```python
from build123d import *

# Parameters (mm, degrees)
F2_W     = 914.4
F2_H     = 457.2
F3_DEPTH = 57.15
F5_DEPTH = 53.975
F6_DEPTH = 57.15


# Not quite as in the source:
# - a length typed as a fraction of an inch, garbled in the dataset ("3 / 203.2 mm" for 3/8 in), is restored


with BuildPart() as f3:
    # F2 (on Top) → F3 (new body)
    with BuildSketch(Plane.XY):
        with Locations((457.2, 228.6)):
            Rectangle(F2_W, F2_H)
    extrude(amount=F3_DEPTH)

    # F4 (on face) → F5 (cut)
    with BuildSketch(Plane.XY.offset(57.15)):
        with BuildLine():
            ThreePointArc((47.625, 23.8125), (44.4270821412, 11.8930134592), (35.692262203, 3.175))
            Line((35.692262203, 3.175), (878.707737797, 3.175))
            ThreePointArc((878.707737797, 3.175), (873.749519773, 40.650480227), (911.225, 35.692262203))
            Line((911.225, 35.692262203), (911.225, 421.507737797))
            ThreePointArc((911.225, 421.507737797), (873.749519773, 416.549519773), (878.707737797, 454.025))
            Line((878.707737797, 454.025), (35.692262203, 454.025))
            ThreePointArc((35.692262203, 454.025), (44.4270821412, 445.3069865408), (47.625, 433.3875))
            ThreePointArc((47.625, 433.3875), (29.9608610621, 410.3824394154), (3.175, 421.507737797))
            Line((3.175, 421.507737797), (3.175, 35.692262203))
            ThreePointArc((3.175, 35.692262203), (29.9608610621, 46.8175605846), (47.625, 23.8125))
        make_face()
    extrude(amount=-F5_DEPTH, mode=Mode.SUBTRACT)

    # F4 (on face) → F6 (cut)
    with BuildSketch(Plane.XY.offset(57.15)):
        with BuildLine():
            Line((11.932737797, 3.175), (3.175, 3.175))
            Line((3.175, 3.175), (3.175, 11.932737797))
            ThreePointArc((3.175, 11.932737797), (0.8074394304, 17.6641388819), (0, 23.8124998841))
            Line((0, 23.8124998841), (0, 0))
            Line((0, 0), (23.8125, 0))
            ThreePointArc((23.8125, 0), (17.6641389379, 0.8074394154), (11.932737797, 3.175))
        make_face()
        with BuildLine():
            Line((3.175, 11.932737797), (3.175, 3.175))
            Line((3.175, 3.175), (11.932737797, 3.175))
            ThreePointArc((11.932737797, 3.175), (6.974519773, 6.974519773), (3.175, 11.932737797))
        make_face()
        with BuildLine():
            ThreePointArc((3.175, 23.8125001882), (9.2195837367, 9.2195838698), (23.8125, 3.175))
            ThreePointArc((23.8125, 3.175), (38.4054161967, 9.2195838033), (44.45, 23.8125))
            ThreePointArc((44.45, 23.8125), (23.8125000941, 44.45), (3.175, 23.8125001882))
        make_face()
        with BuildLine():
            ThreePointArc((23.8124998376, 454.025), (9.2195837458, 447.9804161393), (3.175, 433.3875))
            ThreePointArc((3.175, 433.3875), (23.8125, 412.75), (44.45, 433.3875))
            ThreePointArc((44.45, 433.3875), (38.4054161393, 447.9804162542), (23.8124998376, 454.025))
        make_face()
        with BuildLine():
            Line((3.175, 454.025), (3.175, 445.267262203))
            ThreePointArc((3.175, 445.267262203), (6.974519773, 450.225480227), (11.932737797, 454.025))
            Line((11.932737797, 454.025), (3.175, 454.025))
        make_face()
        with BuildLine():
            Line((0, 457.2), (0, 433.3875))
            ThreePointArc((0, 433.3875), (0.8074394154, 439.5358610621), (3.175, 445.267262203))
            Line((3.175, 445.267262203), (3.175, 454.025))
            Line((3.175, 454.025), (11.932737797, 454.025))
            ThreePointArc((11.932737797, 454.025), (17.6641390246, 456.3925606078), (23.8125001795, 457.2))
            Line((23.8125001795, 457.2), (0, 457.2))
        make_face()
        with BuildLine():
            ThreePointArc((902.467262203, 454.025), (907.425480227, 450.225480227), (911.225, 445.267262203))
            Line((911.225, 445.267262203), (911.225, 454.025))
            Line((911.225, 454.025), (902.467262203, 454.025))
        make_face()
        with BuildLine():
            ThreePointArc((911.225, 445.267262203), (913.5925605846, 439.5358610621), (914.4, 433.3875))
            Line((914.4, 433.3875), (914.4, 457.2))
            Line((914.4, 457.2), (890.5875, 457.2))
            ThreePointArc((890.5875, 457.2), (896.7358610621, 456.3925605846), (902.467262203, 454.025))
            Line((902.467262203, 454.025), (911.225, 454.025))
            Line((911.225, 454.025), (911.225, 445.267262203))
        make_face()
        with BuildLine():
            ThreePointArc((890.5875, 454.025), (875.9945838033, 418.7945838033), (911.225, 433.3875))
            ThreePointArc((911.225, 433.3875), (905.1804161967, 447.9804161967), (890.5875, 454.025))
        make_face()
        with BuildLine():
            ThreePointArc((911.225, 11.932737797), (907.425480227, 6.974519773), (902.467262203, 3.175))
            Line((902.467262203, 3.175), (911.225, 3.175))
            Line((911.225, 3.175), (911.225, 11.932737797))
        make_face()
        with BuildLine():
            ThreePointArc((902.467262203, 3.175), (896.7358610621, 0.8074394154), (890.5875, 0))
            Line((890.5875, 0), (914.4, 0))
            Line((914.4, 0), (914.4, 23.8125))
            ThreePointArc((914.4, 23.8125), (913.5925605846, 17.6641389379), (911.225, 11.932737797))
            Line((911.225, 11.932737797), (911.225, 3.175))
            Line((911.225, 3.175), (902.467262203, 3.175))
        make_face()
        with BuildLine():
            ThreePointArc((911.225, 23.8125), (875.9945838033, 38.4054161967), (890.5875, 3.175))
            ThreePointArc((890.5875, 3.175), (905.1804161967, 9.2195838033), (911.225, 23.8125))
        make_face()
    extrude(amount=-F6_DEPTH, mode=Mode.SUBTRACT)


solid = f3.part
```
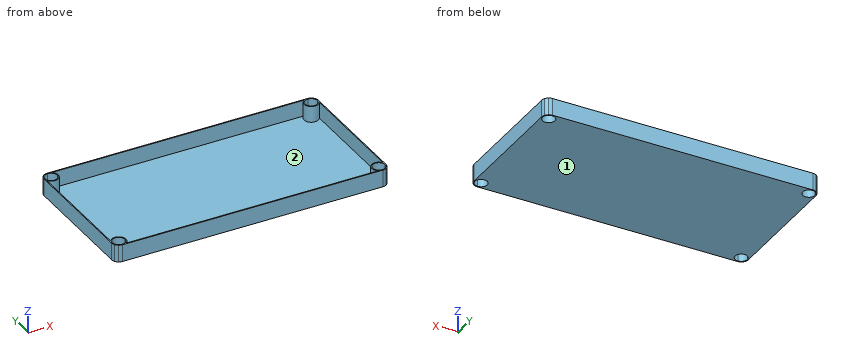
Design review of the part built by this model. Coordinates are the model's own, in mm. Face numbers are marked on the shaded views. Give positions to 0.01 mm unless a question says otherwise; leave off trailing zeros. Order: outer loops, then holes, each group sorted by start corner. A loop starts at its lowest first (then second) coordinate and runs counter-clockwise, first axis right, second up. Notation, with made-up numbers: (56.5, -22) -> (78.5, -22) arc R32 ccw to (78.5, 6) -> close; hole circle Ø11 at (29, -16). An arc over 180 degrees is marked (long way). Write each question's results on one line, items separated by ' | '. Start each with the question number.
Q1. For pin 1 (2 mm diameter, centred on x = 658, y = 315.5, fed in from +Z) (3 decimals), flat-tipped, find the tip position at first contact; note if it passes through.
Q2. Add section A-A on y = 226.5. Give the boundary of the cut face in (x, z) (3 decimals), and give its area (3 significant figures).
Q3. Mouldability with a two-part tool opening along Y and no side actions: class the marked faces 1 and 2 as +Y half, -Y half, draft (parallel to the pull), parting line (faces both ways), or undercut.
Q4. Add section B-B on x = 185. Give the boundary of the cut face in (y, z) (3 decimals).
Q5. Add section C-C on z = 44.5. State how many separate pieces and enclosed holes the cut face has, and give its area (3 significant figures).
Q6. Wall thickness on L1, parallel to Y at x = 357, z = 19 (3 decimals); L2, parallel to X at y = 256, z = 18 (3 decimals); L3, parallel to X at y = 425, z = 36: over which ranges is each line inside the solid? List them lowest first. Write a range as from..to.
Found:
1) pin 1: stops at z = 3.175
2) outline: (0, 0) -> (914.4, 0) -> (914.4, 57.15) -> (911.225, 57.15) -> (911.225, 3.175) -> (3.175, 3.175) -> (3.175, 57.15) -> (0, 57.15) -> close | area: 3,250 mm2
3) face 1: draft | face 2: undercut
4) outline: (0, 0) -> (457.2, 0) -> (457.2, 57.15) -> (454.025, 57.15) -> (454.025, 3.175) -> (3.175, 3.175) -> (3.175, 57.15) -> (0, 57.15) -> close
5) separate pieces: 1 | enclosed holes: 5 | area: 9,670 mm2
6) L1: y = 0..3.175, 454.025..457.2 | L2: x = 0..3.175, 911.225..914.4 | L3: x = 0..4.96, 42.67..46.1, 868.3..871.73, 909.44..914.4
